Source: three-view drawing plus pictorial views. Frame: mm from the lowest corner of the part. A direction names the side the tool comes from. Round coordinates to 2 decimals unless told otherwise and drop trailing zeros. Loops run counter-clockwise (first coordinate to the right, second up) from the corner with the lowest first, then second, coordinate; pieces in that order, holes last. Notation, with made-up numbers: M -3.5,24.25 L 36.5,24.25 A16 cw 36.5,28.25 Z; hole C 34.5,52 d9. An arc over 180 degrees is marked long. Return JSON: item names as keys, results as strings. Group by question number.
1) Access query for the marked faces 1 and 2. Directions: +Z, -Z, +X, -X, +Y, -Y. A direction counts if a zero-diameter tool reaches every point of the face in a straight line with its end or side. Return the directions, or none.
2) Mould query, pull axis Y, two halves, no side actions, for the marked faces 3, 4 and 5. Classes: +Y half, -Y half, draft (parallel to the pull), parting line (faces both ways), or undercut.
3) Material intervals for line 1 (Y direction, x = 3.5, z = 6); line 2 (Y direction, x = 1.5, z = 11); line 3 (Z direction, x = 1.5, y = 1.75), sorted ascending. Write a range as from..to.
4) Section B-B (z = 11.5). Output: boundary loops of the cut face in (x, y).
5) Section C-C (x = 7). Output: boundary loops of the cut face in (y, z).
6) Contact query for flat-ended pins moving along their axis: P1, Ø4, axis at x = 6.5, y = 3.5, coming from the -Z side; P2, Ø3, axis at x = 2.5, z = 6.5, coming from the +Y side. Output: stop coordinate, or through.
7) Section A-A (y = 6). Output: boundary loops of the cut face in (x, z).
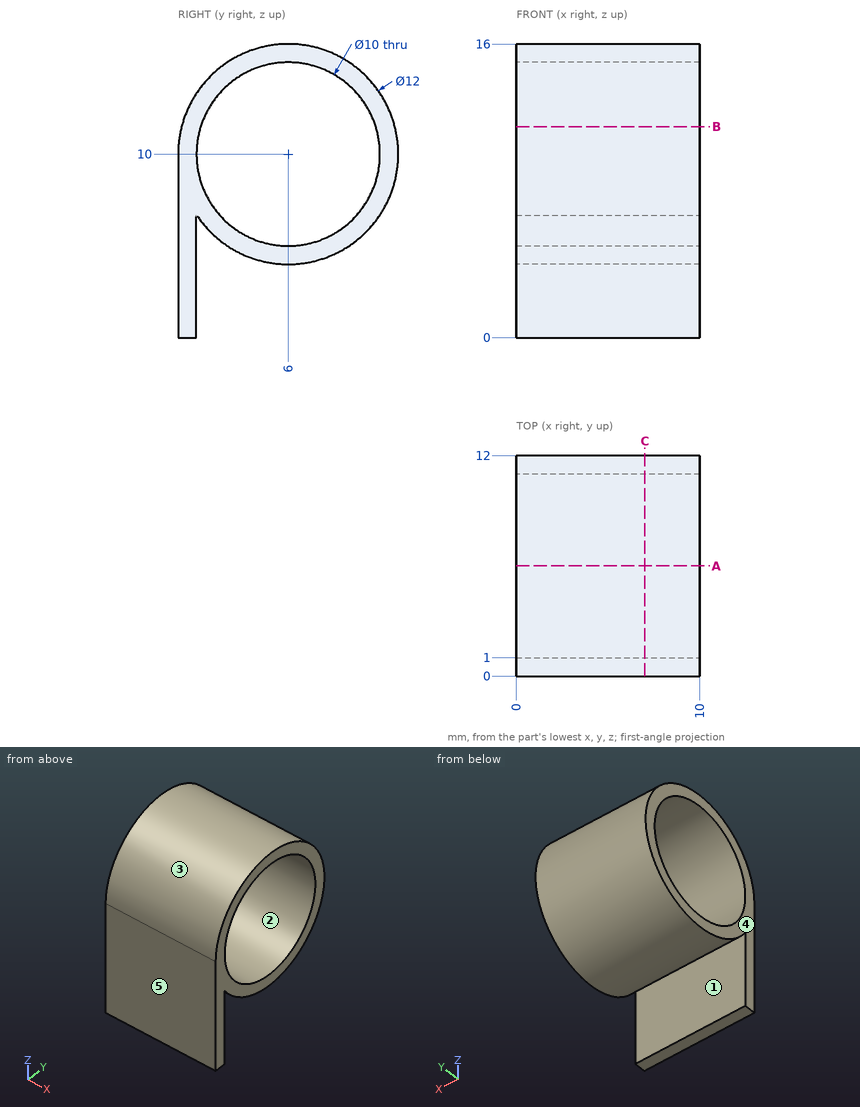
Returned:
{
 "1": {"face 1": "-Z, +X, -X", "face 2": "+X, -X"},
 "2": {"face 3": "undercut", "face 4": "draft", "face 5": "-Y half"},
 "3": {"line 1": "y = 0..1, 1.53..3, 9..10.47", "line 2": "y = 0.08..1.1, 10.9..11.92", "line 3": "z = 5.76..7.37, 12.63..14.24"},
 "4": {"outline": "M 0,0.19 L 10,0.19 L 10,1.23 L 0,1.23 Z; M 0,10.77 L 10,10.77 L 10,11.81 L 0,11.81 Z"},
 "5": {"outline": "M 0,0 L 1,0 L 1,6.68 A6 ccw long 0,10 Z; hole C 6,10 d10"},
 "6": {"P1": "stops at z = 4.02", "P2": "stops at y = 11.66"},
 "7": {"outline": "M 0,4 L 10,4 L 10,5 L 0,5 Z; M 0,15 L 10,15 L 10,16 L 0,16 Z"}
}
